Geometry check sheet. Reference: the model listing, model coordinates, mm. A direction names the side the tool comes from. Give positions to 0.01 mm unless a question says otherwise; leave off trailing zeros. Loops run counter-clockwise (first coordinate to the right, second up) from the corner with the lowest first, then second, coordinate; pieces in that order, holes last. Notation, with made-up numbers: (73, 4.25) -> (88, 4.25) arc R28 ccw to (88, 32.25) -> close; hole circle Ø4 at (34, 0). An arc over 180 degrees is marked (long way). Write item = value, one per line. Start each with the question number.
Autodesk Inventor part; units mm, degrees
ref_plane "YZ Plane" through (0, 0, 0) normal (1, 0, 0) x (0, 1, 0)
ref_plane "XZ Plane" through (0, 0, 0) normal (0, 1, 0) x (-1, 0, 0)
ref_plane "XY Plane" through (0, 0, 0) normal (0, 0, 1) x (1, 0, 0)
sketch "Sketch1" plane through (0, 0, 0) normal (0, 0, 1) x (1, 0, 0)
  line L0 (0, 0) -> (-76.2, 76.2)
  line L1 (-76.2, 76.2) -> (76.2, 76.2)
  line L2 (76.2, 76.2) -> (0, 0)
  point P0 (0, 76.2)
  dimension "d0" = 152.4
  dimension "d2" = 76.2
extrude "Extrusion1" add sketch "Sketch1" against normal blind 6.35
sketch "Sketch2" plane through (0, 0, 0) normal (0, 0, 1) x (1, 0, 0)
  line L0 (-76.2, 76.2) -> (76.2, 76.2)
  line L1 (-19.05, 35.56) -> (-19.05, 45.72)
  arc A0 (19.05, 45.72) -> (-19.05, 45.72) centre (0, 45.72) ccw
  line L2 (19.05, 45.72) -> (19.05, 35.56)
  arc A1 (-19.05, 35.56) -> (19.05, 35.56) centre (0, 35.56) ccw
  point P0 (0, 76.2)
  dimension "d5" = 10.16
  dimension "d6" = 19.05
  dimension "d7" = 30.48
extrude "Extrusion2" cut sketch "Sketch2" against normal through all
ref_plane "Work Plane1" through (76.2, 76.2, -3.175) normal (0, 0, -1) x (-1, 0, 0)
properties part number "GE-13020-02" material "Steel"
1) Depth check by flat-ended pin: pin 1 Ø1.5 at (x, z) = (3.5, -2.5) entering from -Y. Enter the tip coordinate at first touch or a pass-through.
2) Draft check along Y on faces 1 (the cylindrical face through (-0.419, 16.515, -3.131)), 2 (the flat face through (-38, 38, -3)), 3 (the flat face through (-6, 67, 0)), 4 (the flat face through (-19.05, 41, -3)). Enter one of: released by +Y, released by -Y, zero draft, split by the parting line, or undercut.
3) Section check C-C (y = 25.5). Enter the section's corners in (x, z).
4) Tool access check on faces 5 (the cylindrical face through (0.419, 64.765, -3.131)), 6 (the flat face through (-6, 67, -6.35)). Record the directions out of +Z, -Z, +X, -X, +Y, -Y that give a thin tool (end or side, any length) a straight path to the whole face; none if there is none.
5) Section check B-B (x = -4). Enter the section's corners in (y, z), plus the area to 3 significant figures.
6) Thickness scan on line 1 (X direction, y = 39, z = -0.5); line 2 (X direction, y = 30.5, z = -6); line 3 (Y direction, x = -17, z = -3.5). Record the ranges inside material, lowest first.
7) Section check A-A (z = -5). Enter the section's corners in (x, y), plus the area to 3 significant figures.
8) Section check D-D (x = -35). Enter the section's corners in (y, z).
Check result:
q1.pin_1 = 2.75
q2.face_1 = undercut
q2.face_2 = released by -Y
q2.face_3 = zero draft
q2.face_4 = undercut
q3.outline = (-25.5, -6.35) -> (-16.18, -6.35) -> (-16.18, 0) -> (-25.5, 0) -> close; (16.18, -6.35) -> (25.5, -6.35) -> (25.5, 0) -> (16.18, 0) -> close
q4.face_5 = +Z, -Z
q4.face_6 = -Z, +X, -X, +Y, -Y
q5.outline = (4, -6.35) -> (16.93, -6.35) -> (16.93, 0) -> (4, 0) -> close; (64.35, -6.35) -> (76.2, -6.35) -> (76.2, 0) -> (64.35, 0) -> close
q5.area = 157 mm2
q6.line_1 = -39 to -19.05, 19.05 to 39
q6.line_2 = -30.5 to -18.37, 18.37 to 30.5
q6.line_3 = 17 to 26.96, 54.32 to 76.2
q7.outline = (-76.2, 76.2) -> (0, 0) -> (76.2, 76.2) -> close; hole (-19.05, 35.56) arc R19.05 ccw to (19.05, 35.56) -> (19.05, 45.72) arc R19.05 ccw to (-19.05, 45.72) -> close
q7.area = 4,280 mm2
q8.outline = (35, -6.35) -> (76.2, -6.35) -> (76.2, 0) -> (35, 0) -> close
